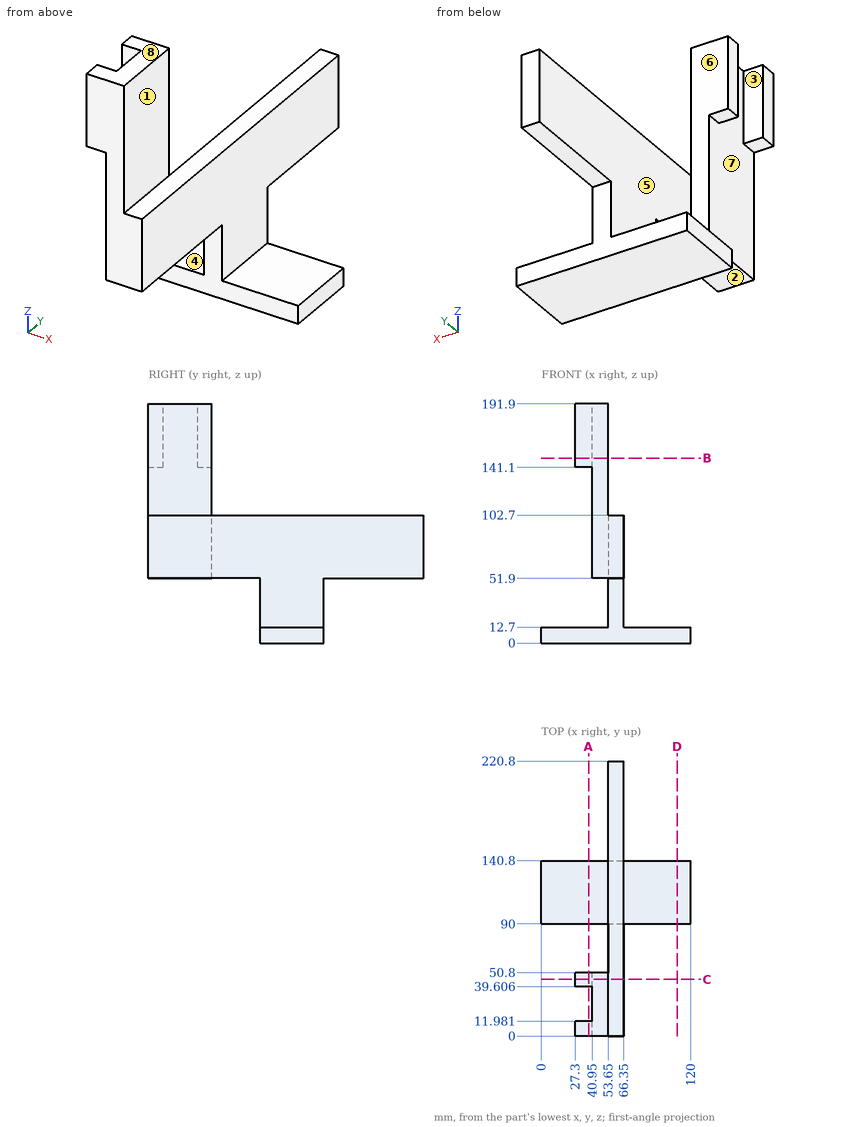
The figure shows three views and two pictorial views of one solid part (mm, origin at its lowest corner). Answer the questions. A direction names the side the tool comes from. Give positions to 0.01 mm unless a question says otherwise; leave off trailing zeros. Order: outer loops, then holes, each group sorted by start corner. A loop starts at its lowest first (then second) coordinate and runs counter-clockwise, first axis right, second up. Notation, with made-up numbers: (43.5, 14) - (92.5, 14) arc R12 ccw to (92.5, 29) - close; hole circle Ø9 at (82.25, 56). An arc over 180 degrees is marked (long way). Answer as CSV lines item,"result".
Q1. Which of the six approach directions +Z, -Z, +X, -X, +Y, -Y give full straight-line access (tool end or side, diameter ignored) to the marked faces 1, 2, 3, 4 and 5?
Answer key:
face 1,"+Z, +X, +Y, -Y"
face 2,"-Z, +X, -X, -Y"
face 3,"+Z, -Z, -X"
face 4,"+Z, -X, +Y, -Y"
face 5,"+Z, -X, +Y"
Q2. Straight lines are drawn through the part: L1, parallel to Y at x = 52.5, z = 151.5; L2, parallel to X at y = 100, z = 34.5; L3, parallel to Y at x = 47.5, z = 10. For each, find the intervals that lie inside material, in ascending order.
Answer key:
L1,"y = 0 to 50.8"
L2,"x = 53.65 to 66.35"
L3,"y = 90 to 140.8"
Q3. Determine the mould class of the marked faces 6, 7 and 8 for opening direction Y: pulls with the +Y half, pulls with the -Y half, needs draft (parallel to the pull), parting line crosses it, or undercut.
Answer key:
face 6,"pulls with the +Y half"
face 7,"undercut"
face 8,"needs draft"
Q4. A cutting plane is placed at D-D, the plane x = 109. Determine the outline of the cut face in (y, z), and give its area (3 significant figures).
Answer key:
outline,"(90, 0) - (140.8, 0) - (140.8, 12.7) - (90, 12.7) - close"
area,"645 mm^2"
Q5. A cutting plane is placed at A-A, the plane x = 38. Determine the outline of the cut face in (y, z), and give its area (3 significant figures).
Answer key:
outline,"(0, 141.1) - (11.98, 141.1) - (11.98, 191.9) - (0, 191.9) - close; (39.61, 141.1) - (50.8, 141.1) - (50.8, 191.9) - (39.61, 191.9) - close; (90, 0) - (140.8, 0) - (140.8, 12.7) - (90, 12.7) - close"
area,"1,820 mm^2"
Q6. A cutting plane is placed at B-B, the plane z = 148.5. Determine the outline of the cut face in (x, y).
Answer key:
outline,"(27.3, 0) - (53.65, 0) - (53.65, 50.8) - (27.3, 50.8) - (27.3, 39.61) - (40.95, 39.61) - (40.95, 11.98) - (27.3, 11.98) - close"
Q7. A cutting plane is placed at C-C, the plane y = 45.5. Determine the outline of the cut face in (x, z).
Answer key:
outline,"(27.3, 141.1) - (40.95, 141.1) - (40.95, 51.9) - (66.35, 51.9) - (66.35, 102.7) - (53.65, 102.7) - (53.65, 191.9) - (27.3, 191.9) - close"
Q8. Each of these flat-tipped pins is pushed along its axis until it touches: pin 1 Ø8 at (x, z) = (42, 146.5) entering from +Y; pin 2 Ø3.5 at (x, y) = (34, 46.5) entering from -Z; pin 3 Ø15 at (x, y) = (97, 110.5) entering from +Z. Where does it stop, or does it pass through?
Answer key:
pin 1,"stops at y = 50.8"
pin 2,"stops at z = 141.1"
pin 3,"stops at z = 12.7"
